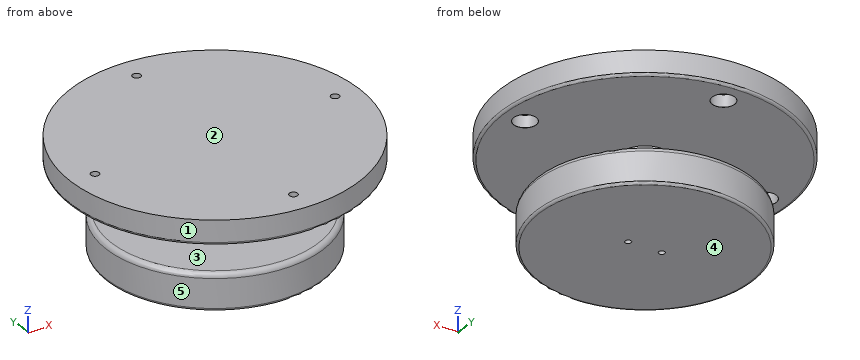
```python
from build123d import *

# Parameters (mm, degrees)
ESQUISSE1_R                                = 45
BOSS_EXTRU_1_DEPTH                         = 15
ESQUISSE3_R                                = 10
BOSS_EXTRU_2_DEPTH                         = 20
ESQUISSE4_R                                = 60
BOSS_EXTRU_3_DEPTH                         = 10
CONG_1_R                                   = 2
CONG_2_R                                   = 1
CONG_3_R                                   = 1
TROU_TARAUD_M31_D                          = 2.5
TROU_TARAUD_M31_DEPTH                      = 12.5
TROU_TARAUD_M31_TIP                        = 0.751075774
CHAMBRAGE_POUR_VIS_T_TE_HEXAGONALE_2_COUNT = 2
CHAMBRAGE_POUR_VIS_T_TE_HEXAGONALE_2_PITCH = 70.710678119
CHAMBRAGE_POUR_VIS_T_TE_HEXAGONALE_3_COUNT = 2
CHAMBRAGE_POUR_VIS_T_TE_HEXAGONALE_3_PITCH = 100
CHAMBRAGE_POUR_VIS_T_TE_HEXAGONALE_4_COUNT = 2
CHAMBRAGE_POUR_VIS_T_TE_HEXAGONALE_4_PITCH = 70.710678119


with BuildPart() as part:
    # Esquisse1 → Boss.-Extru.1 (new body)
    with BuildSketch(Plane.XY):
        Circle(ESQUISSE1_R)
    extrude(amount=BOSS_EXTRU_1_DEPTH)

    # Esquisse3 → Boss.-Extru.2 (add)
    with BuildSketch(Plane.XY.offset(15)):
        Circle(ESQUISSE3_R)
    extrude(amount=BOSS_EXTRU_2_DEPTH)

    # Esquisse4 → Boss.-Extru.3 (add)
    with BuildSketch(Plane.XY.offset(35)):
        Circle(ESQUISSE4_R)
    extrude(amount=BOSS_EXTRU_3_DEPTH)

    # Congé1
    cong_1_edges = [part.edges().sort_by_distance(p)[0] for p in [
        (-45, 0, 15),
    ]]
    fillet(cong_1_edges, radius=CONG_1_R)

    # Congé2
    cong_2_edges = [part.edges().sort_by_distance(p)[0] for p in [
        (-60, 0, 35),
    ]]
    fillet(cong_2_edges, radius=CONG_2_R)

    # Congé3
    cong_3_edges = [part.edges().sort_by_distance(p)[0] for p in [
        (-45, 0, 0),
    ]]
    fillet(cong_3_edges, radius=CONG_3_R)

    # Trou taraudé M31
    with Locations(Plane(origin=(-7, 0, 0), x_dir=(-1, 0, 0), z_dir=(0, 0, -1))):
        with Locations((0, 0), (-14, 0)):
            Hole(TROU_TARAUD_M31_D / 2, depth=TROU_TARAUD_M31_DEPTH)
            with Locations((0, 0, -(TROU_TARAUD_M31_DEPTH + TROU_TARAUD_M31_TIP / 2))):  # 118° drill point
                Cone(0, TROU_TARAUD_M31_D / 2, TROU_TARAUD_M31_TIP, mode=Mode.SUBTRACT)

    # Esquisse9 → Chambrage pour vis à tête hexagonale M31 (revolve, cut)
    with BuildSketch(Plane(origin=(0, 50, 35), x_dir=(0, 1, 0), z_dir=(1, 0, 0))):
        Polygon((0, 0), (0, 10), (1.7, 10), (1.7, 5), (4.6755, 5), (4.6755, 0.025), (4.7005, 0), align=None)
    chambrage_pour_vis_t_te_hexagonale_m31 = revolve(axis=Axis((0, 50, 28.65), (0, 0, 1)), mode=Mode.SUBTRACT)

    # Chambrage pour vis _ t_te hexagonale 2: Chambrage pour vis à tête hexagonale M31 ×2
    with Locations(*[Vector(0.707106781, -0.707106781, 0) * (i * CHAMBRAGE_POUR_VIS_T_TE_HEXAGONALE_2_PITCH) for i in range(1, CHAMBRAGE_POUR_VIS_T_TE_HEXAGONALE_2_COUNT)]):
        add(chambrage_pour_vis_t_te_hexagonale_m31, mode=Mode.SUBTRACT)

    # Chambrage pour vis _ t_te hexagonale 3: Chambrage pour vis à tête hexagonale M31 ×2
    with Locations(*[(0, -i * CHAMBRAGE_POUR_VIS_T_TE_HEXAGONALE_3_PITCH, 0) for i in range(1, CHAMBRAGE_POUR_VIS_T_TE_HEXAGONALE_3_COUNT)]):
        add(chambrage_pour_vis_t_te_hexagonale_m31, mode=Mode.SUBTRACT)

    # Chambrage pour vis _ t_te hexagonale 4: Chambrage pour vis à tête hexagonale M31 ×2
    with Locations(*[Vector(-0.707106781, -0.707106781, 0) * (i * CHAMBRAGE_POUR_VIS_T_TE_HEXAGONALE_4_PITCH) for i in range(1, CHAMBRAGE_POUR_VIS_T_TE_HEXAGONALE_4_COUNT)]):
        add(chambrage_pour_vis_t_te_hexagonale_m31, mode=Mode.SUBTRACT)


solid = part.part
```
Geometry check sheet. Reference: the model listing, model coordinates, mm. Face numbers are marked on the shaded views. A direction names the side the tool comes from. Round coordinates to 2 decimals unless told otherwise and drop trailing zeros. Loops run counter-clockwise (first coordinate to the right, second up) from the corner with the lowest first, then second, coordinate; pieces in that order, holes last. Notation, with made-up numbers: M -5,-31.5 L 14,-31.5 A16 cw 14,-0.5 Z; hole C 88.25,-23 d9. An arc over 180 degrees is marked long. Return JSON: item names as keys, results as strings. Group by question number.
(1) Mould release check, pull along Z, two halves, no side actions. Record for the marked faces 1, 2 and 3: pulls with the +Z half, pulls with the -Z half, needs draft (parallel to the pull), parting line crosses it, or undercut.
(2) Section check A-A, the plane z = 9. Enter the section's corners in (x, y).
(3) Set-up check for the marked faces 4 and 5: record each of +Z, -Z, +X, -X, +Y, -Y from which the full face is reachable in a straight line by a thin tool's end or side.
(4) Go/stop test with flat-tipped pins: pin 1 (6 mm diameter, centred on y = 6.5, z = 8, fed in from -X); pin 2 (11 mm diameter, centred on x = 0, y = -50, fed in from -Z); pin 3 (1.5 mm diameter, centred on x = 35, z = 36, fed in from -Y). Record where each tip stops, or that it passes through.
(5) Section check B-B, the plane z = 17. Enter the section's corners in (x, y).
(6) Scan lines: line 1 along Y through (x, z) = (0, 42.3); line 2 along Y through (x, z) = (0, 38.8); line 3 along Z through (x, y) = (-24, -2). Record each from-to range of solid material in increasing order. Write a range as [from, to].
Data:
{
 "1": {"face 1": "needs draft", "face 2": "pulls with the +Z half", "face 3": "undercut"},
 "2": {"outline": "C 0,0 d90; hole C -7,0 d2.5; hole C 7,0 d2.5"},
 "3": {"face 4": "-Z, +X, -X, +Y, -Y", "face 5": "-Z"},
 "4": {"pin 1": "x = -44.86", "pin 2": "z = 0.13", "pin 3": "y = -49.26"},
 "5": {"outline": "C 0,0 d20"},
 "6": {"line 1": "[-60, -51.7], [-48.3, 48.3], [51.7, 60]", "line 2": "[-60, -54.68], [-45.32, 45.32], [54.68, 60]", "line 3": "[0, 15], [35, 45]"}
}
